Part model, mm, in its own coordinate system. Coordinates: 2 decimals unless noted, no trailing zeros. Order: outer loops, then holes, each group sorted by start corner. A loop starts at its lowest first (then second) coordinate and runs counter-clockwise, first axis right, second up.
from build123d import *

# Parameters (mm, degrees)
F1_DEPTH = 19.05
F2_DEPTH = 3.175
F3_DEPTH = 3.175


with BuildPart() as f1:
    # F0 (on Top) → F1 (new body)
    with BuildSketch(Plane.XY):
        with BuildLine():
            ThreePointArc((3.175, 0), (2.2450640303, 2.2450640303), (0, 3.175))
            Line((0, 3.175), (0, 0))
            Line((0, 0), (3.175, 0))
        make_face()
        with BuildLine():
            Line((0, 0), (0, 3.175))
            ThreePointArc((0, 3.175), (-2.2450640303, 2.2450640303), (-3.175, 0))
            Line((-3.175, 0), (0, 0))
        make_face()
        with BuildLine():
            ThreePointArc((-3.175, 0), (-2.2450640303, -2.2450640303), (0, -3.175))
            Line((0, -3.175), (0, 0))
            Line((0, 0), (-3.175, 0))
        make_face()
        with BuildLine():
            Line((0, 0), (0, -3.175))
            ThreePointArc((0, -3.175), (2.2450640303, -2.2450640303), (3.175, 0))
            Line((3.175, 0), (0, 0))
        make_face()
    extrude(amount=F1_DEPTH)

    # F0 (on Top) → F2 (join)
    with BuildSketch(Plane.XY):
        with BuildLine():
            Line((26.9875, 0), (65.0875, 0))
            ThreePointArc((65.0875, 0), (46.0238126205, 46.0238126205), (0, 65.0875))
            Line((0, 65.0875), (0, 3.175))
            ThreePointArc((0, 3.175), (2.2450640303, 2.2450640303), (3.175, 0))
            Line((3.175, 0), (23.8125, 0))
            ThreePointArc((23.8125, 0), (25.4, 1.5875), (26.9875, 0))
        make_face()
        with BuildLine():
            ThreePointArc((0, -65.0875), (46.0238126205, -46.0238126205), (65.0875, 0))
            Line((65.0875, 0), (26.9875, 0))
            ThreePointArc((26.9875, 0), (25.4, -1.5875), (23.8125, 0))
            Line((23.8125, 0), (3.175, 0))
            ThreePointArc((3.175, 0), (2.2450640303, -2.2450640303), (0, -3.175))
            Line((0, -3.175), (0, -65.0875))
        make_face()
        with BuildLine():
            Line((0, 3.175), (0, 65.0875))
            ThreePointArc((0, 65.0875), (-46.0238126205, 46.0238126205), (-65.0875, 0))
            Line((-65.0875, 0), (-26.9875, 0))
            ThreePointArc((-26.9875, 0), (-25.4, 1.5875), (-23.8125, 0))
            Line((-23.8125, 0), (-3.175, 0))
            ThreePointArc((-3.175, 0), (-2.2450640303, 2.2450640303), (0, 3.175))
        make_face()
        with BuildLine():
            ThreePointArc((-65.0875, 0), (-46.0238126205, -46.0238126205), (0, -65.0875))
            Line((0, -65.0875), (0, -3.175))
            ThreePointArc((0, -3.175), (-2.2450640303, -2.2450640303), (-3.175, 0))
            Line((-3.175, 0), (-23.8125, 0))
            ThreePointArc((-23.8125, 0), (-25.4, -1.5875), (-26.9875, 0))
            Line((-26.9875, 0), (-65.0875, 0))
        make_face()
    extrude(amount=F2_DEPTH)

    # F3 (add): a face of the model
    f3_faces = [f1.faces().sort_by_distance(p)[0] for p in [
        (0, 0, 0),
    ]]
    extrude(f3_faces, amount=F3_DEPTH)


solid = f1.part
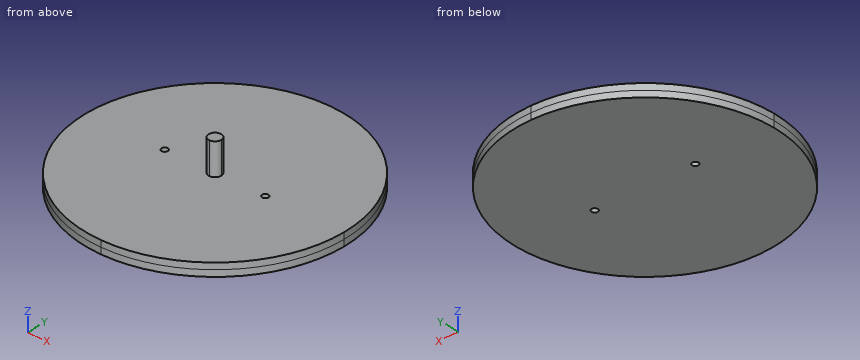
Q1. Pin check, flat tips, straight feed: pin 1 Ø5 at (x, y) = (-22.5, 26) entering from +Z (3 decimals); pin 2 Ø3 at (x, y) = (25.4, 0) entering from +Z; pin 3 Ø6 at (x, z) = (-38, -0.5) entering from +Y; pin 4 Ø10 at (y, z) = (52, 4) entering from +X. Stop position of each tip, or through.
Results list:
pin 1: stops at z = 3.175
pin 2: passes through
pin 3: stops at y = 54.88
pin 4: stops at x = 44.95
Q2. Cut at A-A on x = -25.4. Write the cut outline in (y, z) (1 decimal).
Results list:
outline: (-59.9, -3.2) - (-1.6, -3.2) - (-1.6, 3.2) - (-59.9, 3.2) - close; (1.6, -3.2) - (59.9, -3.2) - (59.9, 3.2) - (1.6, 3.2) - close
Q3. Wall check: line 1 along Z through (x, y) = (-33.5, 15.5) (3 decimals); line 2 along Y through (x, z) = (-25.4, -0.95); line 3 along Y through (x, z) = (0.5, 2). Give the ranges that are in metal, low to high.
Results list:
line 1: z = -3.175 to 3.175
line 2: y = -59.93 to -1.59, 1.59 to 59.93
line 3: y = -65.09 to 65.09
Q4. Cut at C-C on y = 11. Write the cut outline in (x, z) (3 decimals).
Results list:
outline: (-64.151, -3.175) - (64.151, -3.175) - (64.151, 3.175) - (-64.151, 3.175) - close
Q5. Cut at B-B on z = 15.75. Write the cut outline in (x, y) (3 decimals), and give its area (3 significant figures).
Results list:
outline: circle Ø6.35 at (0, 0)
area: 31.7 mm2
